Build history of the part. All positions in model axes, mm. Face numbers are marked on the shaded views. A direction names the side the tool comes from. Give positions to 0.01 mm unless a question says otherwise; leave off trailing zeros. Write each loop counter-clockwise with the first axis right and the second up, starting at its lowest first coordinate (ties: lowest second). Pieces come first, ordered by that corner, then holes.
from build123d import *

# Parameters (mm, degrees)
ESQUISSE1_R        = 1.25
BOSS_EXTRU_1_DEPTH = 6


with BuildPart() as part:
    # Esquisse1 → Boss.-Extru.1 (new body)
    with BuildSketch(Plane.XY):
        with BuildLine():
            Line((14.75, 2.5), (-5.25, 2.5))
            Line((-5.25, 2.5), (-5.25, -7.5))
            Line((-5.25, -7.5), (10.956846109, -7.5))
            Line((10.956846109, -7.5), (10.956846109, -7.7709826))
            Line((10.956846109, -7.7709826), (-1.611734821, -11.948666512))
            ThreePointArc((-1.611734821, -11.948666512), (-5.055755597, -12.442812593), (-1.611966598, -12.938571387))
            Line((-1.611966598, -12.938571387), (14.75, -7.5))
            Line((14.75, -7.5), (14.75, 2.5))
        make_face()
        Circle(ESQUISSE1_R, mode=Mode.SUBTRACT)
        with Locations((9.5, 0)):
            Circle(ESQUISSE1_R, mode=Mode.SUBTRACT)
    extrude(amount=BOSS_EXTRU_1_DEPTH)


solid = part.part
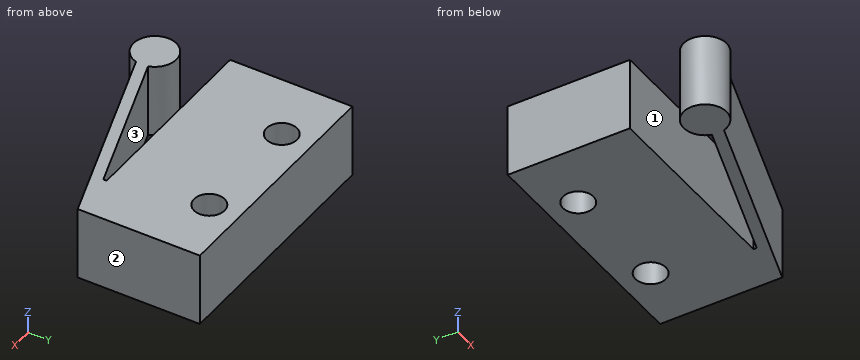
(1) Drop flat-ended pins along their axis: pin 1 (1 mm diameter, centred on x = 4.5, z = 5, fed in from -Y); pin 2 (1.8 mm diameter, centred on x = 0, z = 1.5, fed in from -Y). Give the stop position or say it passes through.
(2) Saw through at A-A, the plane y = 0. List the corners of the cut face in (x, z), plus the area to 3 significant figures.
(3) Saw through at C-C, the plane x = 9.5. List the corners of the cut face in (y, z), plus the area to 3 significant figures.
(4) Saw through at D-D, the plane y = -11.5. List the corners of the cut face in (x, z).
(5) Saw through at B-B, the plane z = 1.8. List the corners of the cut face in (x, y), plus the area to 3 significant figures.
(6) 3-axis set-ups, long thin cutter, end or side, ignore diameter. For the marked faces 1, 2 and 3: which of +Z, -Z, +X, -X, +Y, -Y reach the whole face in a straight line?
(7) Probe line 1 (Y direction, x = 0.25, z = 1.1); line 2 (Y direction, x = -1, z = 4.9); line 3 (X direction, y = 0.5, z = 3.1). List the from-to ranges inside material, lowest first.
Computed values:
1. pin 1: stops at y = -11.07
1. pin 2: stops at y = -12.7
2. outline: (-5.25, 0) - (-1.25, 0) - (-1.25, 6) - (-5.25, 6) - close; (1.25, 0) - (8.25, 0) - (8.25, 6) - (1.25, 6) - close; (10.75, 0) - (14.75, 0) - (14.75, 6) - (10.75, 6) - close
2. area: 90.0 mm2
3. outline: (-9.25, 0) - (-8.26, 0) - (-8.26, 6) - (-9.25, 6) - close; (-7.5, 0) - (-1.25, 0) - (-1.25, 6) - (-7.5, 6) - close; (1.25, 0) - (2.5, 0) - (2.5, 6) - (1.25, 6) - close
3. area: 50.9 mm2
4. outline: (-4.78, 0) - (-1.82, 0) - (-1.82, 6) - (-4.78, 6) - close; (-0.26, 0) - (2.72, 0) - (2.72, 6) - (-0.26, 6) - close
5. outline: (-5.25, -7.5) - (10.96, -7.5) - (10.96, -7.77) - (-1.61, -11.95) arc R1.76 ccw (long way) to (-1.61, -12.94) - (14.75, -7.5) - (14.75, 2.5) - (-5.25, 2.5) - close; hole circle Ø2.5 at (0, 0); hole circle Ø2.5 at (9.5, 0)
5. area: 215 mm2
6. face 1: +Z, -Z, -X
6. face 2: +Z, -Z, +X, +Y, -Y
6. face 3: +Z, -Z
7. line 1: y = -12.32 to -11.33, -7.5 to -1.22, 1.22 to 2.5
7. line 2: y = -12.74 to -11.75, -7.5 to -0.75, 0.75 to 2.5
7. line 3: x = -5.25 to -1.15, 1.15 to 8.35, 10.65 to 14.75
